from build123d import *

# Parameters (mm, degrees)
SALIENTE_EXTRUIR1_DEPTH      = 6
CROQUIS2_W                   = 6
CROQUIS2_H                   = 30
SALIENTE_EXTRUIR2_DEPTH      = 6
SALIENTE_EXTRUIR2_DEPTH_BACK = 96
CORTAR_EXTRUIR1_REACH        = 8
CROQUIS3_R                   = 1.5
CROQUIS3_R_2                 = 10.9
CROQUIS3_R_3                 = 3.9
REDONDEO2_R                  = 10


with BuildPart() as part:
    # Croquis1 → Saliente-Extruir1 (new body)
    with BuildSketch(Plane.XY):
        Polygon((15, -25), (45, -25), (45, 25), (-45, 25), (-45, -25), (-15, -25), (-15, -45), (15, -45), align=None)
    extrude(amount=SALIENTE_EXTRUIR1_DEPTH)

    # Croquis2 → Saliente-Extruir2 (add, two sides)
    with BuildSketch(Plane.ZY.offset(45)) as saliente_extruir2_sk:
        with Locations((3, 0)):
            Rectangle(CROQUIS2_W, CROQUIS2_H)
    extrude(amount=SALIENTE_EXTRUIR2_DEPTH)
    extrude(saliente_extruir2_sk.sketch, amount=-SALIENTE_EXTRUIR2_DEPTH_BACK)

    # Croquis3 → Cortar-Extruir1 (cut, up to next)
    with BuildSketch(Plane.XY.offset(6), mode=Mode.PRIVATE) as cortar_extruir1_sk1:
        with Locations((-15.5, 15.5)):
            Circle(CROQUIS3_R)
    cortar_extruir1_tool1 = extrude(cortar_extruir1_sk1.sketch, amount=-CORTAR_EXTRUIR1_REACH, mode=Mode.PRIVATE) & part.part
    add(cortar_extruir1_tool1.solids().sort_by_distance((-15.5, 15.5, 6))[0], mode=Mode.SUBTRACT)
    # Croquis3 → Cortar-Extruir1 (cut, up to next)
    with BuildSketch(Plane.XY.offset(6), mode=Mode.PRIVATE) as cortar_extruir1_sk2:
        with Locations((15.5, 15.5)):
            Circle(CROQUIS3_R)
    cortar_extruir1_tool2 = extrude(cortar_extruir1_sk2.sketch, amount=-CORTAR_EXTRUIR1_REACH, mode=Mode.PRIVATE) & part.part
    add(cortar_extruir1_tool2.solids().sort_by_distance((15.5, 15.5, 6))[0], mode=Mode.SUBTRACT)
    # Croquis3 → Cortar-Extruir1 (cut, up to next)
    with BuildSketch(Plane.XY.offset(6), mode=Mode.PRIVATE) as cortar_extruir1_sk3:
        with Locations((15.5, -15.5)):
            Circle(CROQUIS3_R)
    cortar_extruir1_tool3 = extrude(cortar_extruir1_sk3.sketch, amount=-CORTAR_EXTRUIR1_REACH, mode=Mode.PRIVATE) & part.part
    add(cortar_extruir1_tool3.solids().sort_by_distance((15.5, -15.5, 6))[0], mode=Mode.SUBTRACT)
    # Croquis3 → Cortar-Extruir1 (cut, up to next)
    with BuildSketch(Plane.XY.offset(6), mode=Mode.PRIVATE) as cortar_extruir1_sk4:
        with Locations((-15.5, -15.5)):
            Circle(CROQUIS3_R)
    cortar_extruir1_tool4 = extrude(cortar_extruir1_sk4.sketch, amount=-CORTAR_EXTRUIR1_REACH, mode=Mode.PRIVATE) & part.part
    add(cortar_extruir1_tool4.solids().sort_by_distance((-15.5, -15.5, 6))[0], mode=Mode.SUBTRACT)
    # Croquis3 → Cortar-Extruir1 (cut, up to next)
    with BuildSketch(Plane.XY.offset(6), mode=Mode.PRIVATE) as cortar_extruir1_sk5:
        Circle(CROQUIS3_R_2)
    cortar_extruir1_tool5 = extrude(cortar_extruir1_sk5.sketch, amount=-CORTAR_EXTRUIR1_REACH, mode=Mode.PRIVATE) & part.part
    add(cortar_extruir1_tool5.solids().sort_by_distance((0, 0, 6))[0], mode=Mode.SUBTRACT)
    # Croquis3 → Cortar-Extruir1 (cut, up to next)
    with BuildSketch(Plane.XY.offset(6), mode=Mode.PRIVATE) as cortar_extruir1_sk6:
        with Locations((0, -35)):
            Circle(CROQUIS3_R_3)
    cortar_extruir1_tool6 = extrude(cortar_extruir1_sk6.sketch, amount=-CORTAR_EXTRUIR1_REACH, mode=Mode.PRIVATE) & part.part
    add(cortar_extruir1_tool6.solids().sort_by_distance((0, -35, 6))[0], mode=Mode.SUBTRACT)

    # Redondeo2
    redondeo2_edges = [part.edges().sort_by_distance(p)[0] for p in [
        (15, -45, 3),
        (-15, -45, 3),
    ]]
    fillet(redondeo2_edges, radius=REDONDEO2_R)


solid = part.part
The model under review builds one solid part; all positions refer to its coordinate system, in mm. A direction names the side the tool comes from. Give positions to 0.01 mm unless a question says otherwise; leave off trailing zeros. Order: outer loops, then holes, each group sorted by start corner. A loop starts at its lowest first (then second) coordinate and runs counter-clockwise, first axis right, second up. Notation, with made-up numbers: (40.25, -21) -> (97.25, -21) arc R11 cw to (97.25, -15) -> close; hole circle Ø5 at (80.5, 24). An arc over 180 degrees is marked (long way). Write item = value, one per line. Start each with the question number.
(1) Take a section at D-D (x = 43). Write out the cut boundary in (y, z).
(2) Take a section at A-A (y = 0). Write out the cut boundary in (x, z).
(3) Draft analysis for pull direction Y (two halves, no side actions). For faces 1 (the flat face through (45, -20, 3)), 2 (the cylindrical face through (12.15, -41.99, 3.04)), 3 (the cylindrical face through (1.8, -38.46, 3.04)), state which applies: +Y half, -Y half, draft (parallel to the pull), parting line (faces both ways), or undercut.
(4) Take a section at C-C (x = 0). Write out the cut boundary in (y, z), plus the area to 3 significant figures.
(5) For pin 1 Ø3 at (x, z) = (-24, 4) entering from -Y; pin 2 Ø1.8 at (x, z) = (-49.5, 2) entering from +Y; pin 3 Ø3 at (y, z) = (-34, 1) entering from +X; pin 4 Ø12 at (x, y) = (-1.5, -24.5) entering from -Z, all flat-tipped, find the tip position at first contact; note any pin that passes through.
(6) Tool access review of faces 4 (the flat face through (48, 15, 3)), 5 (the flat face through (-15, -30, 3)), 6 (the flat face through (30, -25, 3)): name each direction out of +Z, -Z, +X, -X, +Y, -Y from which nothing blocks a thin tool from reaching the whole face with its end or side.
(7) Take a section at B-B (z = 2.25). Write out the cut boundary in (x, y), plus the area to 3 significant figures.
(8) For L1, parallel to Y at x = -15.5, z = 1.9; L2, parallel to X at y = -0.5, z = 1.55; L3, parallel to X at y = -19, z = 4.8, list the stretches that pass through material, from the lowest coordinate up. Write a range as from..to.
Returned:
q1.outline = (-25, 0) -> (25, 0) -> (25, 6) -> (-25, 6) -> close
q2.outline = (-51, 0) -> (-10.9, 0) -> (-10.9, 6) -> (-51, 6) -> close; (10.9, 0) -> (51, 0) -> (51, 6) -> (10.9, 6) -> close
q3.face_1 = draft
q3.face_2 = -Y half
q3.face_3 = undercut
q4.outline = (-45, 0) -> (-38.9, 0) -> (-38.9, 6) -> (-45, 6) -> close; (-31.1, 0) -> (-10.9, 0) -> (-10.9, 6) -> (-31.1, 6) -> close; (10.9, 0) -> (25, 0) -> (25, 6) -> (10.9, 6) -> close
q4.area = 242 mm²
q5.pin_1 = -25
q5.pin_2 = 15
q5.pin_3 = 15
q5.pin_4 = 0
q6.face_4 = +Z, -Z, +X, +Y
q6.face_5 = +Z, -Z, -X, -Y
q6.face_6 = +Z, -Z, +X, -Y
q7.outline = (-51, -15) -> (-45, -15) -> (-45, -25) -> (-15, -25) -> (-15, -35) arc R10 ccw to (-5, -45) -> (5, -45) arc R10 ccw to (15, -35) -> (15, -25) -> (45, -25) -> (45, -15) -> (51, -15) -> (51, 15) -> (45, 15) -> (45, 25) -> (-45, 25) -> (-45, 15) -> (-51, 15) -> close; hole circle Ø3 at (-15.5, -15.5); hole circle Ø3 at (-15.5, 15.5); hole circle Ø21.8 at (0, 0); hole circle Ø7.8 at (0, -35); hole circle Ø3 at (15.5, -15.5); hole circle Ø3 at (15.5, 15.5)
q7.area = 4,970 mm²
q8.L1 = -25..-17, -14..14, 17..25
q8.L2 = -51..-10.89, 10.89..51
q8.L3 = -45..45
